Model file for the job. Use its own axes, mm. Give positions to 0.01 mm unless a question says otherwise; leave off trailing zeros. Loops run counter-clockwise (first coordinate to the right, second up) from the corner with the lowest first, then second, coordinate; pieces in that order, holes last. Notation, with made-up numbers: M 44.25,-12.75 L 90.25,-12.75 A9 ccw 90.25,-6.75 Z; hole C 85,26 d9. An arc over 180 degrees is marked long. Answer in a Markdown table with one row per item.
```python
from build123d import *

# Parameters (mm, degrees)
EXTRUDE_1_DEPTH     = 400
CUT_EXTRUDE_1_DEPTH = 21
CUT_EXTRUDE_2_DEPTH = 21


with BuildPart() as part:
    # Эскиз1 → Бобышка-Вытянуть1 (new body)
    with BuildSketch(Plane.XY):
        with BuildLine():
            Line((-7.5, 12.5), (-7.5, -7.5))
            Line((-7.5, -7.5), (12.5, -7.5))
            Line((12.5, -7.5), (12.5, -4.7))
            ThreePointArc((12.5, -4.7), (12.148528137, -3.851471863), (11.3, -3.5))
            Line((11.3, -3.5), (0, -3.5))
            ThreePointArc((0, -3.5), (-2.474873734, -2.474873734), (-3.5, 0))
            Line((-3.5, 0), (-3.5, 11.3))
            ThreePointArc((-3.5, 11.3), (-3.851471863, 12.148528137), (-4.7, 12.5))
            Line((-4.7, 12.5), (-7.5, 12.5))
        make_face()
    extrude(amount=EXTRUDE_1_DEPTH)

    # Эскиз4 → Вырез-Вытянуть1 (cut, through all)
    with BuildSketch(Plane.XZ.offset(7.5)):
        Polygon((-7.5, 0), (12.5, 0), (12.5, 34.641016151), align=None)
    extrude(amount=-CUT_EXTRUDE_1_DEPTH, mode=Mode.SUBTRACT)

    # Эскиз5 → Вырез-Вытянуть2 (cut, through all)
    with BuildSketch(Plane.XZ.offset(7.5)):
        Polygon((12.5, 400), (-7.5, 400), (12.5, 365.358983849), align=None)
    extrude(amount=-CUT_EXTRUDE_2_DEPTH, mode=Mode.SUBTRACT)


solid = part.part
```
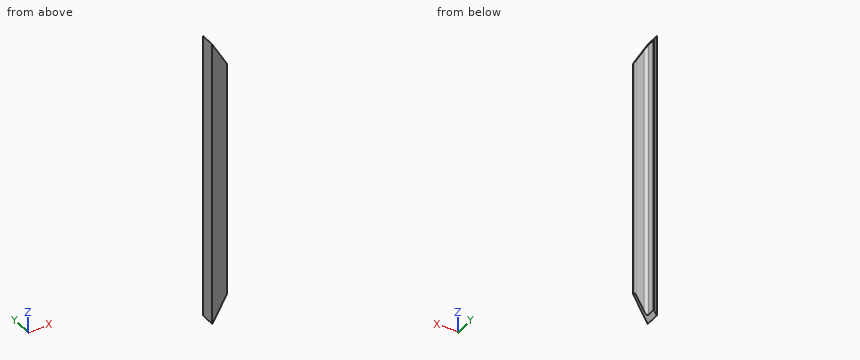
(1) Wall check: L1, parallel to X at y = 9.25, z = 241; L2, parallel to Y at x = -4.5, z = 150.5. Give the ranges that are in metal, low to high.
Established:
| item | result |
|---|---|
| L1 | x = -7.5 to -3.5 |
| L2 | y = -7.5 to 12.48 |
(2) Saw through at B-B, the plane y = 7.5. Give the cut face in (x, z), and give its area (3 significant figures).
Established:
| item | result |
|---|---|
| outline | M -7.5,0 L -3.5,6.93 L -3.5,393.07 L -7.5,400 Z |
| area | 1,570 mm2 |
(3) Flat gauge pins, fed straight in: P1, Ø6, axis at x = -3.5, y = -2.5, coming from the +Z side; P2, Ø3.5, axis at x = 8, z = 281, coming from the +Y side; P3, Ø10, axis at x = 8, y = -5, coming from the +Z side. Where does each tip first touch, or does it go through?
Established:
| item | result |
|---|---|
| P1 | stops at z = 398.27 |
| P2 | stops at y = -3.5 |
| P3 | stops at z = 381.81 |
(4) Saw through at A-A, the plane z = 354. Give the cut face in (x, y), and give its area (3 significant figures).
Established:
| item | result |
|---|---|
| outline | M -7.5,-7.5 L 12.5,-7.5 L 12.5,-4.7 A1.2 ccw 11.3,-3.5 L 0,-3.5 A3.5 cw -3.5,0 L -3.5,11.3 A1.2 ccw -4.7,12.5 L -7.5,12.5 Z |
| area | 146 mm2 |
(5) Saw through at C-C, the plane x = 3.75. Give the cut face in (y, z).
Established:
| item | result |
|---|---|
| outline | M -7.5,19.49 L -3.5,19.49 L -3.5,380.51 L -7.5,380.51 Z |
